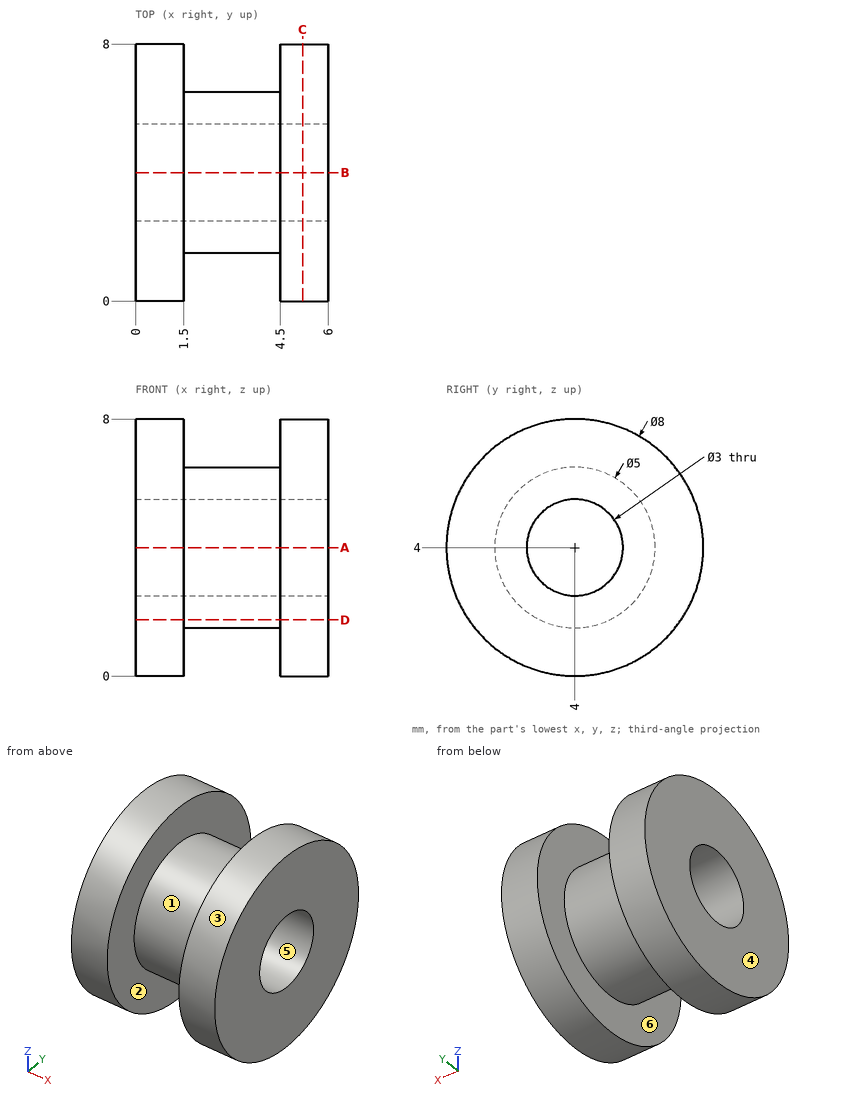
Answer from the drawing. Dimensions are ordinates in mm from the lowest x, y and z of the part. A direction names the side the tool comes from. Give positions to 0.01 mm unless a question says otherwise; leave off trailing zeros. Order: outer loops, then holes, each group sorted by start corner. A loop starts at its lowest first (then second) coordinate and runs counter-clockwise, first axis right, second up. Notation, with made-up numbers: (7, -31) -> (21, -31) arc R19 cw to (21, 6) -> close; hole circle Ø11 at (42.5, -6). An arc over 180 degrees is marked (long way). One line per item, written item: value. Start each with the question number.
(1) The part is cut by section A-A (z = 4). Determine the outline of the cut face in (x, y).
(2) Flat-ended cylindrical pins translate along their axes: P1, Ø1.5, axis at x = 3.5, z = 7, coming from the -Y side; P2, Ø1, axis at x = 3.5, y = 6.5, coming from the -Z side; P3, Ø3, axis at x = 5.5, y = 7, coming from the -Z side. Find the tip coordinate at first contact, or state that the pin passes through.
(3) Straight lines are drawn through the part: L1, parallel to Z at x = 4.3, y = 4; L2, parallel to X at y = 2.25, z = 0.5; L3, parallel to Z at x = 5, y = 5. For each, find the intervals that lie inside material, in ascending order.
(4) The part is cut by section D-D (z = 1.75). Determine the outline of the cut face in (x, y).
(5) For a pull along X with two mould halves and no side action, classify the marked faces 1, 2, 3 and 4 as released by +X, released by -X, zero draft, split by the parting line, or undercut.
(6) A tool of negligible diameter and unlimited length cuts with its end or side. For the marked faces 5 and 6, from which of +Z, -Z, +X, -X, +Y, -Y can it reach the whole face along a straight path? Write none if from no direction.
(7) The part is cut by section C-C (x = 5.2). Determine the outline of the cut face in (y, z).
Taken from the geometry:
1. outline: (0, 0) -> (1.5, 0) -> (1.5, 1.5) -> (4.5, 1.5) -> (4.5, 0) -> (6, 0) -> (6, 2.5) -> (0, 2.5) -> close; (0, 5.5) -> (6, 5.5) -> (6, 8) -> (4.5, 8) -> (4.5, 6.5) -> (1.5, 6.5) -> (1.5, 8) -> (0, 8) -> close
2. P1: y = 2.91
2. P2: z = 2.5
2. P3: z = 0.29
3. L1: 1.5 to 2.5, 5.5 to 6.5
3. L2: 0 to 1.5, 4.5 to 6
3. L3: 0.13 to 2.88, 5.12 to 7.87
4. outline: (0, 0.69) -> (1.5, 0.69) -> (1.5, 2.91) -> (4.5, 2.91) -> (4.5, 0.69) -> (6, 0.69) -> (6, 7.31) -> (4.5, 7.31) -> (4.5, 5.09) -> (1.5, 5.09) -> (1.5, 7.31) -> (0, 7.31) -> close
5. face 1: undercut
5. face 2: undercut
5. face 3: zero draft
5. face 4: released by -X
6. face 5: +X, -X
6. face 6: none
7. outline: circle Ø8 at (4, 4); hole circle Ø3 at (4, 4)
